from build123d import *

# Parameters (mm, degrees)
F0_R     = 20
F1_DEPTH = 15
F2_R     = 18
F3_DEPTH = 13
F4_R     = 3.5
F4_R_2   = 1.5
F5_DEPTH = 16
F8_DEPTH = 10


with BuildPart() as f1:
    # F0 (on Top) → F1 (new body)
    with BuildSketch(Plane.XY):
        Circle(F0_R)
    extrude(amount=F1_DEPTH)

    # F2 (on face) → F3 (cut)
    with BuildSketch(Plane.XY.offset(15)):
        Circle(F2_R)
    extrude(amount=-F3_DEPTH, mode=Mode.SUBTRACT)

    # F4 (on face) → F5 (join)
    with BuildSketch(Plane.XY.offset(2)):
        Circle(F4_R)
        Circle(F4_R_2, mode=Mode.SUBTRACT)
    extrude(amount=F5_DEPTH)

    # F7 (on face) → F8 (cut)
    with BuildSketch(Plane.XY):
        with BuildLine():
            Line((10.0770842302, -8.2639499676), (2.3258358706, -3.7887646407))
            Line((2.3258358706, -3.7887646407), (2.3258358706, -12.8589859232))
            Line((2.3258358706, -12.8589859232), (4.0292034895, -17.5432471122))
            ThreePointArc((4.0292034895, -17.5432471122), (8.8280697184, -15.6864650271), (12.9055203458, -12.5478103509))
            Line((12.9055203458, -12.5478103509), (10.0770842302, -8.2639499676))
        make_face()
        with BuildLine():
            Line((-2.1182484925, -12.8589859232), (-2.1182484925, -3.9086152693))
            Line((-2.1182484925, -3.9086152693), (-9.9732905411, -8.4437259106))
            Line((-9.9732905411, -8.4437259106), (-13.1782959193, -12.261016135))
            ThreePointArc((-13.1782959193, -12.261016135), (-9.1708423498, -15.4885651561), (-4.4139623529, -17.450413644))
            Line((-4.4139623529, -17.450413644), (-2.1182484925, -12.8589859232))
        make_face()
        with BuildLine():
            Line((-12.1953327227, -4.5950359556), (-4.4440843631, -0.1198506286))
            Line((-4.4440843631, -0.1198506286), (-12.2991264117, 4.4152600127))
            Line((-12.2991264117, 4.4152600127), (-17.2074994088, 5.2822309772))
            ThreePointArc((-17.2074994088, 5.2822309772), (-17.9989120683, 0.197899871), (-17.3194826987, -4.9026032931))
            Line((-17.3194826987, -4.9026032931), (-12.1953327227, -4.5950359556))
        make_face()
        with BuildLine():
            Line((-10.0770842302, 8.2639499676), (-2.3258358706, 3.7887646407))
            Line((-2.3258358706, 3.7887646407), (-2.3258358706, 12.8589859232))
            Line((-2.3258358706, 12.8589859232), (-4.0292034895, 17.5432471122))
            ThreePointArc((-4.0292034895, 17.5432471122), (-8.8280697184, 15.6864650271), (-12.9055203458, 12.5478103509))
            Line((-12.9055203458, 12.5478103509), (-10.0770842302, 8.2639499676))
        make_face()
        with BuildLine():
            Line((2.1182484925, 12.8589859232), (2.1182484925, 3.9086152693))
            Line((2.1182484925, 3.9086152693), (9.9732905411, 8.4437259106))
            Line((9.9732905411, 8.4437259106), (13.1782959193, 12.261016135))
            ThreePointArc((13.1782959193, 12.261016135), (9.1708423498, 15.4885651561), (4.4139623529, 17.450413644))
            Line((4.4139623529, 17.450413644), (2.1182484925, 12.8589859232))
        make_face()
        with BuildLine():
            Line((12.1953327227, 4.5950359556), (4.4440843631, 0.1198506286))
            Line((4.4440843631, 0.1198506286), (12.2991264117, -4.4152600127))
            Line((12.2991264117, -4.4152600127), (17.2074994088, -5.2822309772))
            ThreePointArc((17.2074994088, -5.2822309772), (17.8007723057, -2.6706750684), (18, 0))
            ThreePointArc((18, 0), (17.8290589849, 2.4748041764), (17.3194826987, 4.9026032931))
            Line((17.3194826987, 4.9026032931), (12.1953327227, 4.5950359556))
        make_face()
    extrude(amount=F8_DEPTH, mode=Mode.SUBTRACT)


solid = f1.part
Part model, mm, in its own coordinate system. A direction names the side the tool comes from. Give positions to 0.01 mm unless a question says otherwise; leave off trailing zeros. Order: outer loops, then holes, each group sorted by start corner. A loop starts at its lowest first (then second) coordinate and runs counter-clockwise, first axis right, second up. Notation, with made-up numbers: (18.25, 6.25) -> (70.25, 6.25) arc R24 ccw to (70.25, 24.25) -> close; hole circle Ø4 at (87, 68). An arc over 180 degrees is marked (long way). Use one line per item in the form item = value.
(1) Tool access for faces 1 (the face through (-8.32, 2.12, 0.99)), 2 (the face through (0, 0, 2)): list every direction of +Z, -Z, +X, -X, +Y, -Y with a clear straight run to the whole face (end or side of a thin tool).
Solution:
face_1 = +Z, -Z
face_2 = +Z
(2) Pull direction Y, two halves, no side cores. Call faces 3 (the face through (14.719, -4.843, 0.986)), 4 (the face through (-4.336, -19.524, 7.395)): +Y half, -Y half, draft (parallel to the pull), parting line (faces both ways), or undercut.
Solution:
face_3 = undercut
face_4 = parting line
(3) Flat gauge pins, fed straight in: P1, Ø0.9, axis at x = -0.5, y = -0.5, coming from the +Z side; P2, Ø2.5, axis at x = 0, y = 0, coming from the -Z side; P3, Ø4, axis at y = -8.5, z = 6, coming from the +X side; P4, Ø3, axis at y = 5, z = 9.5, coming from the +X side. Where does each tip first touch, or does it go through?
Solution:
P1 = 2
P2 = 0
P3 = 18.91
P4 = 19.69
(4) Saw through at B-B (y = -2). Write the cut outline in (x, z).
Solution:
outline = (-19.9, 0) -> (-17.89, 0) -> (-17.89, 15) -> (-19.9, 15) -> close; (-7.7, 0) -> (8.12, 0) -> (8.12, 2) -> (2.87, 2) -> (2.87, 18) -> (-2.87, 18) -> (-2.87, 2) -> (-7.7, 2) -> close; (17.89, 0) -> (19.9, 0) -> (19.9, 15) -> (17.89, 15) -> close
(5) Saw through at A-A (z = 6). Write the cut outline in (x, y).
Solution:
outline = circle Ø40 at (0, 0); circle Ø7 at (0, 0); hole circle Ø36 at (0, 0); hole circle Ø3 at (0, 0)
(6) Saw through at C-C (x = 6.5). Write the cut outline in (y, z), then the cut area to 3 significant figures.
Solution:
outline = (-18.91, 0) -> (-16.79, 0) -> (-16.79, 15) -> (-18.91, 15) -> close; (-6.2, 0) -> (-1.07, 0) -> (-1.07, 2) -> (-6.2, 2) -> close; (1.31, 0) -> (6.44, 0) -> (6.44, 2) -> (1.31, 2) -> close; (16.79, 0) -> (18.91, 0) -> (18.91, 15) -> (16.79, 15) -> close
area = 84.4 mm²
(7) Drill centre lines: line 1 (Y direction, x = 0, z = 13); line 2 (Y direction, x = 17, z = 1.25); line 3 (Z direction, x = 10.5, y = -5). Where is each one in solid material? Low to high. Write a range as from..to.
Solution:
line_1 = -20..-18, -3.5..-1.5, 1.5..3.5, 18..20
line_2 = -10.54..-5.25, 4.88..10.54
line_3 = 0..2
(8) Saw through at D-D (x = 0). Write the cut outline in (y, z).
Solution:
outline = (-20, 0) -> (20, 0) -> (20, 15) -> (18, 15) -> (18, 2) -> (3.5, 2) -> (3.5, 18) -> (1.5, 18) -> (1.5, 2) -> (-1.5, 2) -> (-1.5, 18) -> (-3.5, 18) -> (-3.5, 2) -> (-18, 2) -> (-18, 15) -> (-20, 15) -> close
